from build123d import *

# Parameters (mm, degrees)
F0_W     = 70
F0_H     = 51
F1_DEPTH = 1.5
F2_R     = 1.5
F3_DEPTH = 1.501
F4_W     = 15
F4_H     = 34
F5_DEPTH = 16.5
F6_W     = 10
F6_H     = 4.5
F7_DEPTH = 19


with BuildPart() as f1:
    # F0 (on Top) → F1 (new body)
    with BuildSketch(Plane.XY):
        with Locations((35, 25.5)):
            Rectangle(F0_W, F0_H)
    extrude(amount=F1_DEPTH)

    # F2 (on face) → F3 (cut, through all)
    with BuildSketch(Plane.XY.offset(1.5)):
        with Locations((67, 47.75)):
            Circle(F2_R)
        with Locations((67, 3.25)):
            Circle(F2_R)
        with Locations((3, 47.75)):
            Circle(F2_R)
        with Locations((3, 3.25)):
            Circle(F2_R)
    extrude(amount=-F3_DEPTH, mode=Mode.SUBTRACT)

    # F4 (on face) → F5 (join)
    with BuildSketch(Plane.XY.offset(1.5)):
        with Locations((41.5, 25)):
            Rectangle(F4_W, F4_H)
    extrude(amount=F5_DEPTH)

    # F6 (on face) → F7 (join)
    with BuildSketch(Plane.XY.offset(1.5)):
        with Locations((55, 41.25)):
            Rectangle(F6_W, F6_H)
    extrude(amount=F7_DEPTH)


solid = f1.part
Check sheet for the modelled part. Datum: model origin and axes. Units: mm. A direction names the side the tool comes from. Give positions to 0.01 mm unless a question says otherwise; leave off trailing zeros. Loops run counter-clockwise (first coordinate to the right, second up) from the corner with the lowest first, then second, coordinate; pieces in that order, holes last. Notation, with made-up numbers: M 58,-22 L 112,-22 A6 cw 112,-17 Z; hole C -12.5,50.5 d10. An arc over 180 degrees is marked long. Return JSON: item names as keys, results as strings. Group by question number.
1. Cross-section at A-A on z = 2.75. Record the boundary of the cut face in (x, y).
2. Go/stop test with flat-tipped pins: pin 1 (12 mm diameter, centred on x = 31.5, z = 8, fed in from +Y); pin 2 (6 mm diameter, centred on x = 29.5, y = 38.5, fed in from +Z); pin 3 (4 mm diameter, centred on x = 33.5, y = 30, fed in from +Z). Record where each tip stops, or that it passes through.
3. Cross-section at D-D on x = 54.5. Record the boundary of the cut face in (y, z).
4. Thickness scan on L1, parallel to Y at x = 67, z = 0.4; L2, parallel to X at y = 35, z = 7; L3, parallel to Z at x = 35, y = 38.5. Record the ranges inside material, lowest first.
5. Tool access check on faces 5 (the flat face through (41, 8, 10)), 6 (the flat face through (34, 25, 10)), 7 (the flat face through (41, 42, 10)), 8 (the flat face through (55, 43.5, 11)), 9 (the cylindrical face through (2.675, 46.286, 0.76)). Record the directions out of +Z, -Z, +X, -X, +Y, -Y that give a thin tool (end or side, any length) a straight path to the whole face; none if there is none.
6. Mould release check, pull along X, two halves, no side actions. Record for faces 1 (the flat face through (60, 41, 11)), 2 (the flat face through (55, 39, 11)), 3 (the flat face through (0, 25, 1)), 4 (the cylindrical face through (67.69, 46.42, 0.76)): released by +X, released by -X, zero draft, split by the parting line, or undercut.
7. Cross-section at B-B on y = 47.75. Record the boundary of the cut face in (x, z), plus the area to 3 significant figures.
8. Cross-section at C-C on x = 3. Record the boundary of the cut face in (y, z), plus the area to 3 significant figures.
Return value:
{
 "1": {"outline": "M 34,8 L 49,8 L 49,42 L 34,42 Z; M 50,39 L 60,39 L 60,43.5 L 50,43.5 Z"},
 "2": {"pin 1": "y = 42", "pin 2": "z = 1.5", "pin 3": "z = 18"},
 "3": {"outline": "M 0,0 L 51,0 L 51,1.5 L 43.5,1.5 L 43.5,20.5 L 39,20.5 L 39,1.5 L 0,1.5 Z"},
 "4": {"L1": "0 to 1.75, 4.75 to 46.25, 49.25 to 51", "L2": "34 to 49", "L3": "0 to 18"},
 "5": {"face 5": "+Z, +X, -X, -Y", "face 6": "+Z, -X, +Y, -Y", "face 7": "+Z, -X, +Y", "face 8": "+Z, +X, -X, +Y", "face 9": "+Z, -Z"},
 "6": {"face 1": "released by +X", "face 2": "zero draft", "face 3": "released by -X", "face 4": "undercut"},
 "7": {"outline": "M 0,0 L 1.5,0 L 1.5,1.5 L 0,1.5 Z; M 4.5,0 L 65.5,0 L 65.5,1.5 L 4.5,1.5 Z; M 68.5,0 L 70,0 L 70,1.5 L 68.5,1.5 Z", "area": "96.0 mm^2"},
 "8": {"outline": "M 0,0 L 1.75,0 L 1.75,1.5 L 0,1.5 Z; M 4.75,0 L 46.25,0 L 46.25,1.5 L 4.75,1.5 Z; M 49.25,0 L 51,0 L 51,1.5 L 49.25,1.5 Z", "area": "67.5 mm^2"}
}
